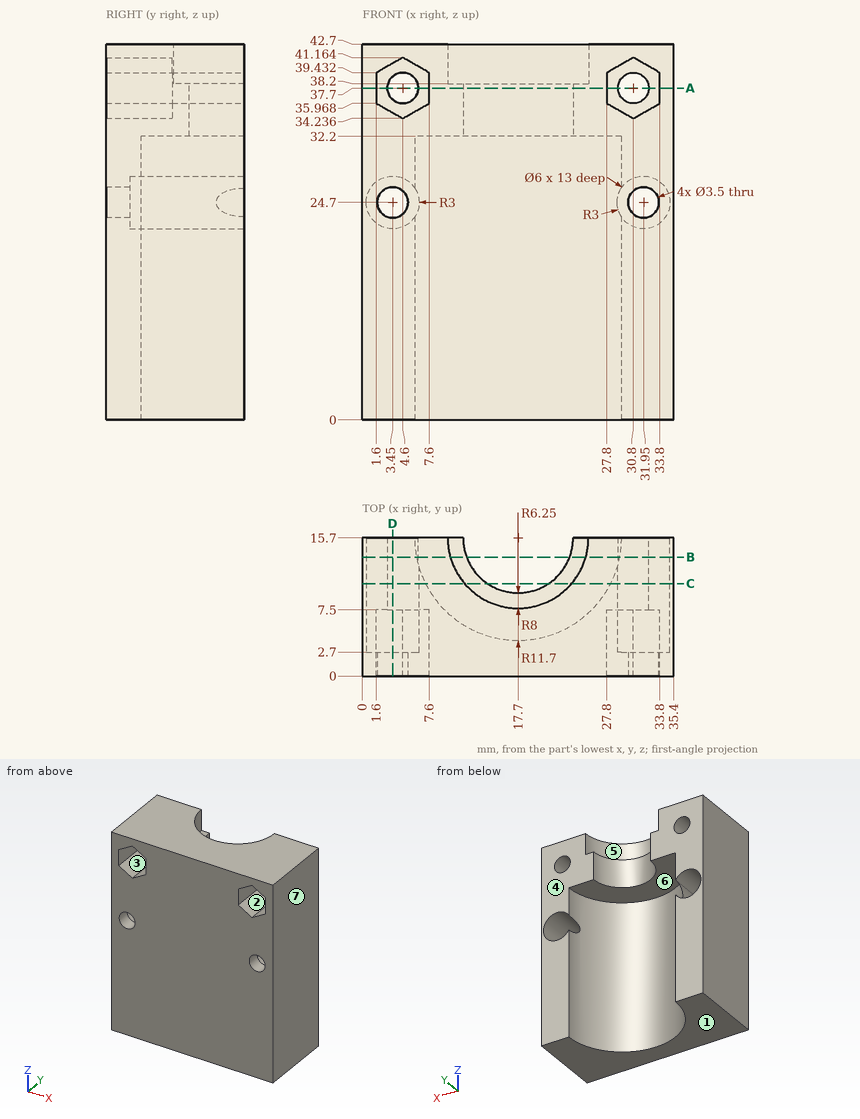
Answer from the drawing. Dimensions are ordinates in mm from the lowest x, y and z of the part. A direction names the side the tool comes from. Round coordinates to 2 decimals unless told otherwise and drop trailing zeros. Loops run counter-clockwise (first coordinate to the right, second up) from the corner with the lowest first, then second, coordinate; pieces in that order, holes last.
1) For a pull along Z with two mould halves and no side action, classify the marked faces 1, 2, 3 and 4 as released by +Z, released by -Z, zero draft, split by the parting line, or undercut.
Outcome:
face 1: released by -Z
face 2: undercut
face 3: undercut
face 4: zero draft
2) A cutting plane is placed at D-D on x = 3.45. Determine the outline of the cut face in (y, z), plus the area to 3 significant figures.
Outcome:
outline: (0, 0) - (15.7, 0) - (15.7, 21.7) - (2.7, 21.7) - (2.7, 22.95) - (0, 22.95) - close; (0, 26.45) - (2.7, 26.45) - (2.7, 27.7) - (15.7, 27.7) - (15.7, 36.38) - (7.5, 36.38) - (7.5, 34.9) - (0, 34.9) - close; (0, 40.5) - (7.5, 40.5) - (7.5, 39.02) - (15.7, 39.02) - (15.7, 42.7) - (0, 42.7) - close
area: 519 mm2
3) Given P1, Ø6, axis at x = 22, y = 9.5, coming from the -Z side; P2, Ø5.5, axis at x = 4.6, z = 37.7, coming from the -Y side; P3, Ø2, axis at x = 3.45, z = 24.7, coming from the -Y side; P4, Ø3, axis at x = 3, z = 24, coming from the +Y side, each flat-ended and moving along its own axis, determine where each tip first touches the part or whether it passes through.
Outcome:
P1: stops at z = 32.2
P2: stops at y = 7.5
P3: passes through
P4: stops at y = 2.7
4) Consider line 1 (Z direction, x = 3.45, y = 1.8); line 2 (X direction, y = 6.5, z = 11); line 3 (Z direction, x = 4.6, y = 11.5). Determine where each line is inside the solid, lowest interval first.
Outcome:
line 1: z = 0 to 22.95, 26.45 to 34.9, 40.5 to 42.7
line 2: x = 0 to 10.47, 24.93 to 35.4
line 3: z = 0 to 21.93, 27.47 to 35.95, 39.45 to 42.7
5) For the marked faces 5, 6 and 7, determine the directions among +Z, -Z, +X, -X, +Y, -Y from which every point of the face is accessible in a straight line to the end or side of a thin tool.
Outcome:
face 5: +Z, +Y
face 6: -Z, +Y
face 7: +Z, -Z, +X, +Y, -Y
6) A cutting plane is placed at A-A on z = 37.7. Determine the outline of the cut face in (x, y), plus the area to 3 significant figures.
Outcome:
outline: (0, 0) - (1.6, 0) - (1.6, 7.5) - (2.85, 7.5) - (2.85, 15.7) - (0, 15.7) - close; (6.35, 7.5) - (7.6, 7.5) - (7.6, 0) - (27.8, 0) - (27.8, 7.5) - (29.05, 7.5) - (29.05, 15.7) - (23.95, 15.7) arc R6.25 cw to (11.45, 15.7) - (6.35, 15.7) - close; (32.55, 7.5) - (33.8, 7.5) - (33.8, 0) - (35.4, 0) - (35.4, 15.7) - (32.55, 15.7) - close
area: 347 mm2
7) A cutting plane is placed at C-C on y = 10.5. Determine the outline of the cut face in (x, z).
Outcome:
outline: (0, 0) - (7.22, 0) - (7.22, 32.2) - (14.23, 32.2) - (14.23, 38.2) - (11.62, 38.2) - (11.62, 42.7) - (0, 42.7) - close; (21.17, 32.2) - (28.18, 32.2) - (28.18, 0) - (35.4, 0) - (35.4, 42.7) - (23.78, 42.7) - (23.78, 38.2) - (21.17, 38.2) - close; hole circle Ø6 at (3.45, 24.7); hole circle Ø3.5 at (4.6, 37.7); hole circle Ø6 at (31.95, 24.7); hole circle Ø3.5 at (30.8, 37.7)
8) A cutting plane is placed at B-B on y = 13.5. Determine the outline of the cut face in (x, z).
Outcome:
outline: (0, 0) - (6.21, 0) - (6.21, 23.52) arc R3 cw (long way) to (6.21, 25.88) - (6.21, 32.2) - (11.85, 32.2) - (11.85, 38.2) - (10.01, 38.2) - (10.01, 42.7) - (0, 42.7) - close; (23.55, 32.2) - (29.19, 32.2) - (29.19, 25.88) arc R3 cw (long way) to (29.19, 23.52) - (29.19, 0) - (35.4, 0) - (35.4, 42.7) - (25.39, 42.7) - (25.39, 38.2) - (23.55, 38.2) - close; hole circle Ø3.5 at (4.6, 37.7); hole circle Ø3.5 at (30.8, 37.7)
